```python
from build123d import *

# Parameters (mm, degrees)
F1_DEPTH = 350


with BuildPart() as f1:
    # F0 (on Top) → F1 (new body)
    with BuildSketch(Plane.XY):
        with BuildLine():
            ThreePointArc((-290, 4), (-288.828427, 1.171573), (-286, 0))
            Line((-286, 0), (-244, 0))
            ThreePointArc((-244, 0), (-241.171573, 1.171573), (-240, 4))
            Line((-240, 4), (-240, 15))
            Line((-240, 15), (-242, 15))
            Line((-242, 15), (-242, 4))
            ThreePointArc((-242, 4), (-242.585786, 2.585786), (-244, 2))
            Line((-244, 2), (-286, 2))
            ThreePointArc((-286, 2), (-287.414214, 2.585786), (-288, 4))
            Line((-288, 4), (-288, 404))
            ThreePointArc((-288, 404), (-287.414214, 405.414214), (-286, 406))
            Line((-286, 406), (286, 406))
            ThreePointArc((286, 406), (287.414214, 405.414214), (288, 404))
            Line((288, 404), (288, 4))
            ThreePointArc((288, 4), (287.414214, 2.585786), (286, 2))
            Line((286, 2), (244, 2))
            ThreePointArc((244, 2), (242.585786, 2.585786), (242, 4))
            Line((242, 4), (242, 15))
            Line((242, 15), (240, 15))
            Line((240, 15), (240, 4))
            ThreePointArc((240, 4), (241.171573, 1.171573), (244, 0))
            Line((244, 0), (286, 0))
            ThreePointArc((286, 0), (288.828427, 1.171573), (290, 4))
            Line((290, 4), (290, 404))
            ThreePointArc((290, 404), (288.828427, 406.828427), (286, 408))
            Line((286, 408), (-286, 408))
            ThreePointArc((-286, 408), (-288.828427, 406.828427), (-290, 404))
            Line((-290, 404), (-290, 4))
        make_face()
    extrude(amount=-F1_DEPTH)


solid = f1.part
```
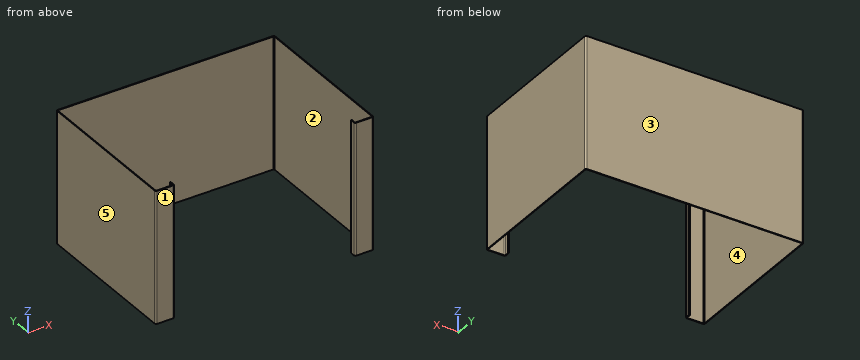
For this review, take the finished solid that the model builds, in its own axes (mm). Face numbers are marked on the shaded views. A direction names the side the tool comes from. Coordinates: 2 decimals unless noted, no trailing zeros. Loops run counter-clockwise (first coordinate to the right, second up) from the corner with the lowest first, then second, coordinate; pieces in that order, holes last. Notation, with made-up numbers: (-14, 83.5) -> (40, 83.5) arc R9 ccw to (40, 97.5) -> close; hole circle Ø1 at (52.25, 71.25). An arc over 180 degrees is marked (long way). Return JSON: item names as keys, results as strings. Group by question number.
(1) Consider section C-C, the plane x = -183.5. Give the boundary of the cut face in (y, z).
(2) To check wall thickness, follow L1, parallel to X at y = 385.5, z = -299; L2, parallel to Y at x = -259.5, z = -247; L3, parallel to Y at x = 225.5, z = -261. State the ranges of each line that lie inside material, in increasing order.
(3) Tool access review of the marked faces 1 and 2: name each direction out of +Z, -Z, +X, -X, +Y, -Y from which nothing blocks a thin tool from reaching the whole face with its end or side.
(4) Consider section A-A, the plane y = 327.5. Give the boundary of the cut face in (x, z).
(5) For pin 1 Ø4 at (x, z) = (53, -168.5) entering from -Y, flat-tipped, find the tip position at first contact; note if it passes through.
(6) Consider section B-B, the plane z = -207.5. Give the boundary of the cut face in (x, y), plus the area to 3 significant figures.
(7) Mouldability with a two-part tool opening along X and no side actions: class the marked faces 3, 4 and 5 as pulls with the +X half, pulls with the -X half, needs draft (parallel to the pull), parting line crosses it, or undercut.
Results below:
{
 "1": {"outline": "(406, -350) -> (408, -350) -> (408, 0) -> (406, 0) -> close"},
 "2": {"L1": "x = -290 to -288, 288 to 290", "L2": "y = 0 to 2, 406 to 408", "L3": "y = 406 to 408"},
 "3": {"face 1": "+Z, -Z, +X, -X, -Y", "face 2": "+Z, -Z"},
 "4": {"outline": "(-290, -350) -> (-288, -350) -> (-288, 0) -> (-290, 0) -> close; (288, -350) -> (290, -350) -> (290, 0) -> (288, 0) -> close"},
 "5": {"pin 1": "stops at y = 406"},
 "6": {"outline": "(-290, 4) arc R4 ccw to (-286, 0) -> (-244, 0) arc R4 ccw to (-240, 4) -> (-240, 15) -> (-242, 15) -> (-242, 4) arc R2 cw to (-244, 2) -> (-286, 2) arc R2 cw to (-288, 4) -> (-288, 404) arc R2 cw to (-286, 406) -> (286, 406) arc R2 cw to (288, 404) -> (288, 4) arc R2 cw to (286, 2) -> (244, 2) arc R2 cw to (242, 4) -> (242, 15) -> (240, 15) -> (240, 4) arc R4 ccw to (244, 0) -> (286, 0) arc R4 ccw to (290, 4) -> (290, 404) arc R4 ccw to (286, 408) -> (-286, 408) arc R4 ccw to (-290, 404) -> close", "area": "3,010 mm2"},
 "7": {"face 3": "needs draft", "face 4": "undercut", "face 5": "pulls with the -X half"}
}
